For this review, use the dimensioned drawing (mm, ordinates from the lowest corner) and the shaded views. Coordinates: 2 decimals unless noted, no trailing zeros. Write each loop counter-clockwise with the first axis right and the second up, starting at its lowest first coordinate (ties: lowest second). Pieces come first, ordered by that corner, then holes. Notation, with made-up numbers: M 42,-9.5 L 70,-9.5 A10 ccw 70,-3.5 Z; hole C -14,-33 d6. An arc over 180 degrees is marked long. One line per question, with ' | ' between items.
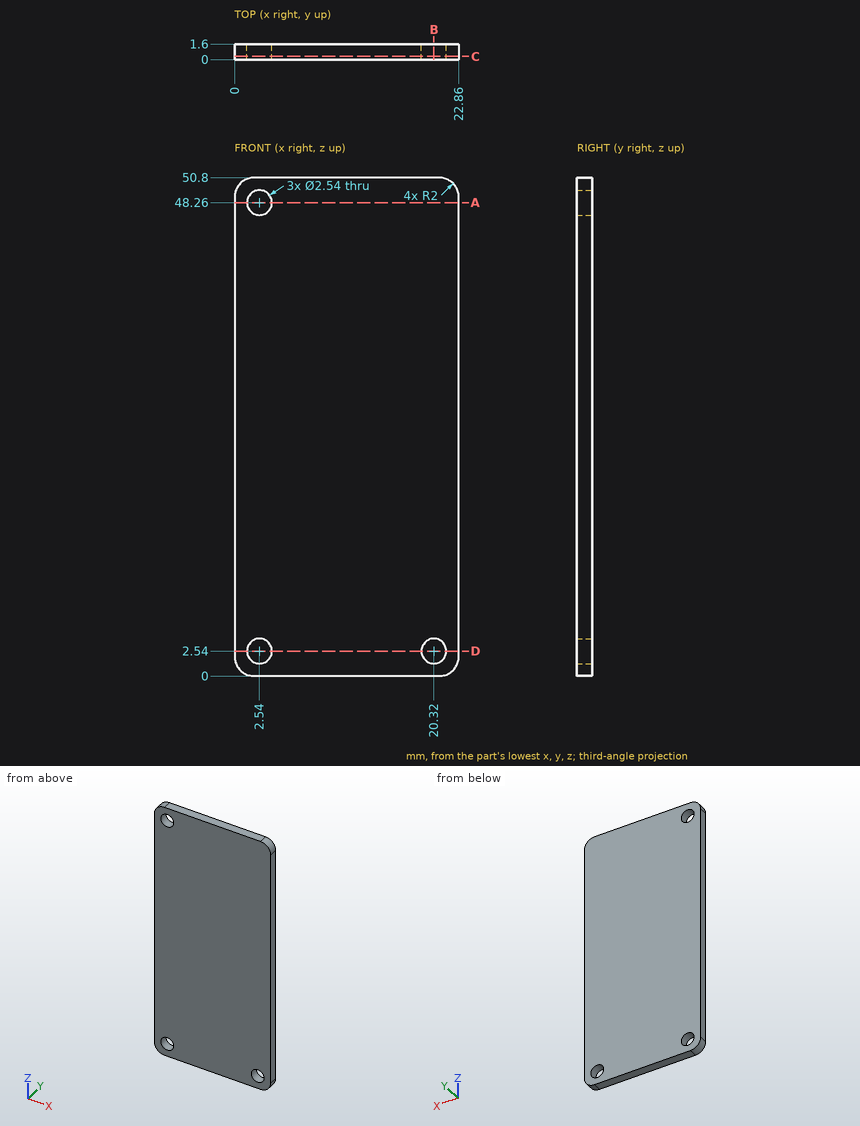
1. To check wall thickness, follow line 1 along Z through (x, y) = (2.54, 1.05); line 2 along Z through (x, y) = (3.5, 0.1); line 3 along Z through (x, y) = (20.32, 1). State the ranges of each line that lie inside material, in increasing order. Write a range as [from, to].
Answer sheet:
line 1: [0, 1.27], [3.81, 46.99], [49.53, 50.8] | line 2: [0, 1.71], [3.37, 47.43], [49.09, 50.8] | line 3: [0, 1.27], [3.81, 50.8]
2. Take a section at A-A (z = 48.26). Write out the cut boundary in (x, y), then the cut area to 3 significant figures.
Answer sheet:
outline: M 0,0 L 1.27,0 L 1.27,1.6 L 0,1.6 Z; M 3.81,0 L 22.86,0 L 22.86,1.6 L 3.81,1.6 Z | area: 32.5 mm^2
3. Take a section at D-D (z = 2.54). Write out the cut boundary in (x, y).
Answer sheet:
outline: M 0,0 L 1.27,0 L 1.27,1.6 L 0,1.6 Z; M 3.81,0 L 19.05,0 L 19.05,1.6 L 3.81,1.6 Z; M 21.59,0 L 22.86,0 L 22.86,1.6 L 21.59,1.6 Z
4. Take a section at C-C (y = 0.35). Write out the cut boundary in (x, z).
Answer sheet:
outline: M 0,2 A2 ccw 2,0 L 20.86,0 A2 ccw 22.86,2 L 22.86,48.8 A2 ccw 20.86,50.8 L 2,50.8 A2 ccw 0,48.8 Z; hole C 2.54,2.54 d2.54; hole C 2.54,48.26 d2.54; hole C 20.32,2.54 d2.54
5. Take a section at B-B (x = 20.32). Write out the cut boundary in (y, z), then the cut area to 3 significant figures.
Answer sheet:
outline: M 0,0 L 1.6,0 L 1.6,1.27 L 0,1.27 Z; M 0,3.81 L 1.6,3.81 L 1.6,50.8 L 0,50.8 Z | area: 77.2 mm^2
